from build123d import *

# Parameters (mm, degrees)
SALIENTE_EXTRUIR2_DEPTH = 4.5


with BuildPart() as part:
    # Croquis1 → Saliente-Extruir2 (new body)
    with BuildSketch(Plane.XY):
        with BuildLine():
            Line((19, 4.5), (-19, 4.5))
            ThreePointArc((-19, 4.5), (-23.5, 0), (-19, -4.5))
            Line((-19, -4.5), (19, -4.5))
            ThreePointArc((19, -4.5), (23.5, 0), (19, 4.5))
        make_face()
        with BuildLine():
            Line((18.75, 2.25), (16.25, 2.25))
            ThreePointArc((16.25, 2.25), (14, 0), (16.25, -2.25))
            Line((16.25, -2.25), (18.75, -2.25))
            ThreePointArc((18.75, -2.25), (21, 0), (18.75, 2.25))
        make_face(mode=Mode.SUBTRACT)
        with BuildLine():
            Line((-16.25, 2.25), (-18.75, 2.25))
            ThreePointArc((-18.75, 2.25), (-21, 0), (-18.75, -2.25))
            Line((-18.75, -2.25), (-16.25, -2.25))
            ThreePointArc((-16.25, -2.25), (-14, 0), (-16.25, 2.25))
        make_face(mode=Mode.SUBTRACT)
    extrude(amount=SALIENTE_EXTRUIR2_DEPTH)


solid = part.part
Geometry check sheet. Reference: the model listing, model coordinates, mm. A direction names the side the tool comes from. Give positions to 0.01 mm unless a question says otherwise; leave off trailing zeros. Write each loop counter-clockwise with the first axis right and the second up, starting at its lowest first coordinate (ties: lowest second). Pieces come first, ordered by that corner, then holes. Notation, with made-up numbers: (42, 4) - (61, 4) arc R13 ccw to (61, 18) - close; hole circle Ø5 at (75, 12). An arc over 180 degrees is marked (long way). Put each result on its own line as item: value.
1. Draft check along Y on faces 1 (the cylindrical face through (-23.5, 0.1, 2.2)), 2 (the flat face through (-17, 2.25, 2)), 3 (the flat face through (0, 4.5, 2)). Enter one of: +Y half, -Y half, draft (parallel to the pull), parting line (faces both ways), or undercut.
Ans:
face 1: parting line
face 2: undercut
face 3: +Y half
2. Sectioned sample at A-A, the plane x = -17.5. Enter the section's corners in (y, z).
Ans:
outline: (-4.5, 0) - (-2.25, 0) - (-2.25, 4.5) - (-4.5, 4.5) - close; (2.25, 0) - (4.5, 0) - (4.5, 4.5) - (2.25, 4.5) - close
3. Set-up check for faces 4 (the flat face through (0, 0, 0)), 5 (the flat face through (18, 2.25, 2)): record each of +Z, -Z, +X, -X, +Y, -Y from which the full face is reachable in a straight line by a thin tool's end or side.
Ans:
face 4: -Z, +X, -X, +Y, -Y
face 5: +Z, -Z
4. Go/stop test with a flat-tipped pin: pin 1 (2 mm diameter, centred on x = 2.5, y = -0.5, fed in from -Z). Record where the tip stops, or that it passes through.
Ans:
pin 1: stops at z = 0
5. Sectioned sample at D-D, the plane y = 1.25. Enter the section's corners in (x, z).
Ans:
outline: (-23.32, 0) - (-20.62, 0) - (-20.62, 4.5) - (-23.32, 4.5) - close; (-14.38, 0) - (14.38, 0) - (14.38, 4.5) - (-14.38, 4.5) - close; (20.62, 0) - (23.32, 0) - (23.32, 4.5) - (20.62, 4.5) - close
6. Thickness scan on line 1 (X direction, y = 0, z = 0.75); line 2 (X direction, y = -1.75, z = 2.95); line 3 (Y direction, x = 17.5, z = 3.3). Record the ranges inside material, lowest first.
Ans:
line 1: x = -23.5 to -21, -14 to 14, 21 to 23.5
line 2: x = -23.15 to -20.16, -14.84 to 14.84, 20.16 to 23.15
line 3: y = -4.5 to -2.25, 2.25 to 4.5
7. Sectioned sample at B-B, the plane z = 1.45. Enter the section's corners in (x, y), plus the area to 3 significant figures.
Ans:
outline: (-19, -4.5) - (19, -4.5) arc R4.5 ccw to (19, 4.5) - (-19, 4.5) arc R4.5 ccw to start; hole (-18.75, -2.25) - (-16.25, -2.25) arc R2.25 ccw to (-16.25, 2.25) - (-18.75, 2.25) arc R2.25 ccw to start; hole (16.25, -2.25) - (18.75, -2.25) arc R2.25 ccw to (18.75, 2.25) - (16.25, 2.25) arc R2.25 ccw to start
area: 351 mm²
8. Sectioned sample at C-C, the plane y = -1.5. Enter the section's corners in (x, z), plus the area to 3 significant figures.
Ans:
outline: (-23.24, 0) - (-20.43, 0) - (-20.43, 4.5) - (-23.24, 4.5) - close; (-14.57, 0) - (14.57, 0) - (14.57, 4.5) - (-14.57, 4.5) - close; (20.43, 0) - (23.24, 0) - (23.24, 4.5) - (20.43, 4.5) - close
area: 156 mm²
